Part print with two shaded views. Sizes in mm from the minimum x, y, z corner. A direction names the side the tool comes from. Give positions to 0.01 mm unless a question says otherwise; leave off trailing zeros. Write each loop counter-clockwise with the first axis right and the second up, starting at its lowest first coordinate (ties: lowest second). Pieces come first, ordered by that corner, then holes. Notation, with made-up numbers: (-34, 59) -> (19, 59) arc R17 ccw to (19, 70) -> close; hole circle Ø6 at (-30, 35.25). An arc over 180 degrees is marked (long way). Answer in a Markdown table with one row per item. Add a question column.
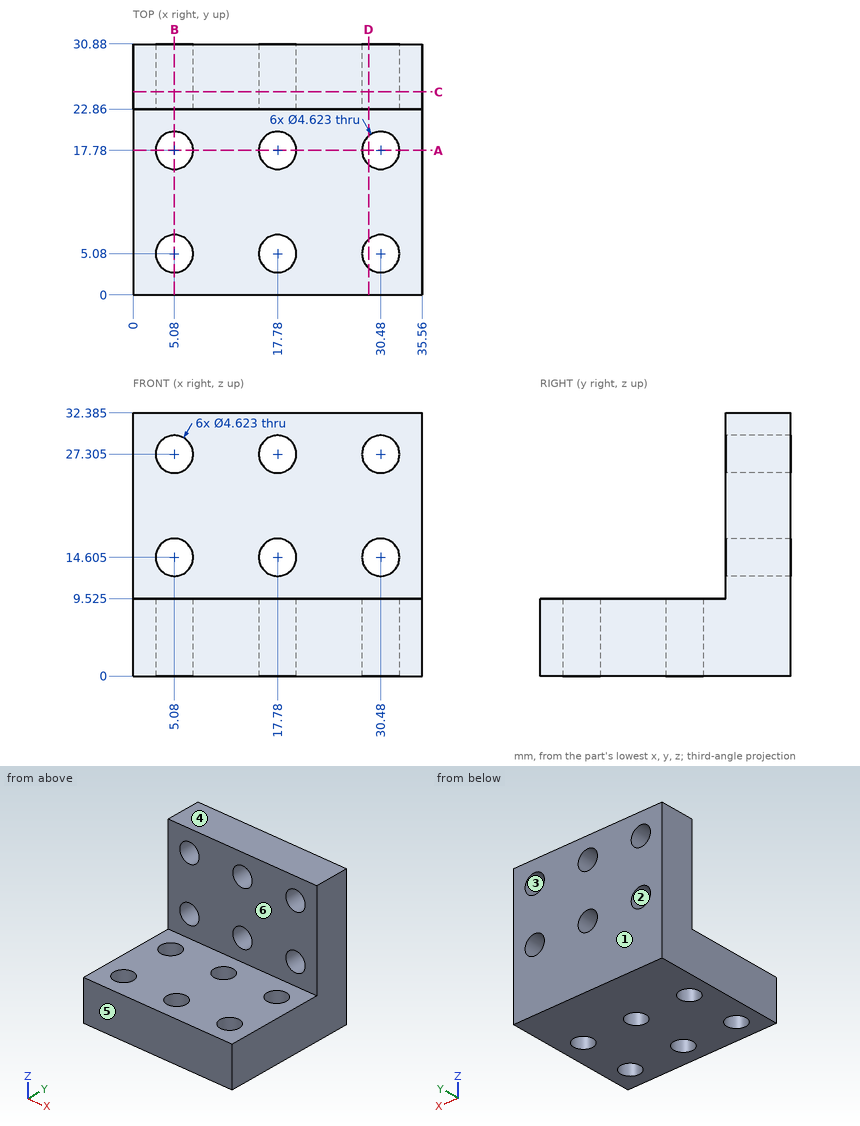
Item 1: Which spindle directions (+Z, -Z, +X, -X, +Y, -Y) get a long thin tool onto all of the face, cutting with end or side? Do the marked faces 5 and 6. Say none if no direction does.
Item 2: Slice it at B-B, the plane x = 5.08. List the corners of the cut face in (y, z) (1 decimal).
Item 3: Probe L1, parallel to Z at x = 30.48, y = 27.25 (1 decimal); L2, parallel to Z at x = 19, y = 26 (1 decimal); L3, parallel to Y at x = 6.5, z = 3. List the from-to ranges inside material, lowest first. Write a range as from..to.
Item 4: Slice it at A-A, the plane y = 17.78. List the corners of the cut face in (x, z) (1 decimal).
Item 5: Mould opens along Z. For the marked faces 1, 2, 3 and 4 say: released by +Z, released by -Z, zero draft, split by the parting line, or undercut.
Item 6: Slice it at C-C, the plane y = 25. List the corners of the cut face in (x, z) (1 decimal), then the cut area to 3 significant figures.
Item 7: Drop flat-ended pins along their axis: pin 1 Ø6 at (x, y) = (17.78, 5.08) entering from +Z (3 decimals); pin 2 Ø7.5 at (x, z) = (30.48, 27.305) entering from -Y. Give the stop position or say it passes through.
Item 8: Slice it at D-D, the plane x = 29. List the corners of the cut face in (y, z) (1 decimal), then the cut area to 3 significant figures.
Answer key:
| question | item | result |
|---|---|---|
| 1 | face 5 | +Z, -Z, +X, -X, -Y |
| 1 | face 6 | +Z, +X, -X, -Y |
| 2 | outline | (0, 0) -> (2.8, 0) -> (2.8, 9.5) -> (0, 9.5) -> close; (7.4, 0) -> (15.5, 0) -> (15.5, 9.5) -> (7.4, 9.5) -> close; (20.1, 0) -> (30.9, 0) -> (30.9, 12.3) -> (22.9, 12.3) -> (22.9, 9.5) -> (20.1, 9.5) -> close; (22.9, 16.9) -> (30.9, 16.9) -> (30.9, 25) -> (22.9, 25) -> close; (22.9, 29.6) -> (30.9, 29.6) -> (30.9, 32.4) -> (22.9, 32.4) -> close |
| 3 | L1 | z = 0..12.3, 16.9..25, 29.6..32.4 |
| 3 | L2 | z = 0..12.6, 16.6..25.3, 29.3..32.4 |
| 3 | L3 | y = 0..3.26, 6.9..15.96, 19.6..30.88 |
| 4 | outline | (0, 0) -> (2.8, 0) -> (2.8, 9.5) -> (0, 9.5) -> close; (7.4, 0) -> (15.5, 0) -> (15.5, 9.5) -> (7.4, 9.5) -> close; (20.1, 0) -> (28.2, 0) -> (28.2, 9.5) -> (20.1, 9.5) -> close; (32.8, 0) -> (35.6, 0) -> (35.6, 9.5) -> (32.8, 9.5) -> close |
| 5 | face 1 | zero draft |
| 5 | face 2 | undercut |
| 5 | face 3 | undercut |
| 5 | face 4 | released by +Z |
| 6 | outline | (0, 0) -> (35.6, 0) -> (35.6, 32.4) -> (0, 32.4) -> close; hole circle Ø4.6 at (5.1, 14.6); hole circle Ø4.6 at (5.1, 27.3); hole circle Ø4.6 at (17.8, 14.6); hole circle Ø4.6 at (17.8, 27.3); hole circle Ø4.6 at (30.5, 14.6); hole circle Ø4.6 at (30.5, 27.3) |
| 6 | area | 1,050 mm² |
| 7 | pin 1 | stops at z = 9.525 |
| 7 | pin 2 | stops at y = 22.86 |
| 8 | outline | (0, 0) -> (3.3, 0) -> (3.3, 9.5) -> (0, 9.5) -> close; (6.9, 0) -> (16, 0) -> (16, 9.5) -> (6.9, 9.5) -> close; (19.6, 0) -> (30.9, 0) -> (30.9, 12.8) -> (22.9, 12.8) -> (22.9, 9.5) -> (19.6, 9.5) -> close; (22.9, 16.4) -> (30.9, 16.4) -> (30.9, 25.5) -> (22.9, 25.5) -> close; (22.9, 29.1) -> (30.9, 29.1) -> (30.9, 32.4) -> (22.9, 32.4) -> close |
| 8 | area | 353 mm² |
